```python
from build123d import *

# Parameters (mm, degrees)
EXTRUDE_1_DEPTH     = 3
EXTRUDE_2_DEPTH     = 5.8
SKETCH_3_W          = 1.5
SKETCH_3_H          = 2
SKETCH_3_R          = 0.85
EXTRUDE_3_DEPTH     = 3
CUT_EXTRUDE_1_DEPTH = 8.8


with BuildPart() as part:
    # 草图1 → 凸台-拉伸1 (new body)
    with BuildSketch(Plane.XY):
        Polygon((0, 0), (-28.5, 0), (-28.5, 15), (-8.5, 15), (-8.5, 24.333), (0, 24.333), align=None)
    extrude(amount=EXTRUDE_1_DEPTH)

    # 草图2 → 凸台-拉伸2 (add)
    with BuildSketch(Plane.XY.offset(3)):
        Polygon((-12, 15), (-9.228718708, 10.2), (0, 10.2), (0, 0), (-28.5, 0), (-28.5, 15), align=None)
    extrude(amount=EXTRUDE_2_DEPTH)

    # 草图3 → 凸台-拉伸3 (add)
    with BuildSketch(Plane.XY.offset(3)):
        with Locations((-0.75, 19.6)):
            Rectangle(SKETCH_3_W, SKETCH_3_H)
        with Locations((-0.75, 14.5)):
            Rectangle(SKETCH_3_W, SKETCH_3_H)
        with Locations(Location((-3.5, 13.8, 0), (0, 0, 180))):
            Circle(SKETCH_3_R)
        with Locations(Location((-3.5, 20.3, 0), (0, 0, 180))):
            Circle(SKETCH_3_R)
    extrude(amount=EXTRUDE_3_DEPTH)

    # 草图5 → 切除-拉伸1 (cut)
    with BuildSketch(Plane.XY.offset(8.8)):
        with BuildLine():
            ThreePointArc((-20.5, 7.5), (-22.5, 9.5), (-24.5, 7.5))
            Line((-24.5, 7.5), (-20.5, 7.5))
        make_face()
        with BuildLine():
            Line((-20.5, 7.5), (-24.5, 7.5))
            ThreePointArc((-24.5, 7.5), (-22.5, 5.5), (-20.5, 7.5))
        make_face()
        with BuildLine():
            ThreePointArc((-10.5, 7.5), (-12.5, 9.5), (-14.5, 7.5))
            Line((-14.5, 7.5), (-10.5, 7.5))
        make_face()
        with BuildLine():
            Line((-10.5, 7.5), (-14.5, 7.5))
            ThreePointArc((-14.5, 7.5), (-12.5, 5.5), (-10.5, 7.5))
        make_face()
    extrude(amount=-CUT_EXTRUDE_1_DEPTH, mode=Mode.SUBTRACT)


solid = part.part
```
Work out the finished part from the listing and answer in its coordinate system (mm). A direction names the side the tool comes from. Give positions to 0.01 mm unless a question says otherwise; leave off trailing zeros. Write each loop counter-clockwise with the first axis right and the second up, starting at its lowest first coordinate (ties: lowest second). Pieces come first, ordered by that corner, then holes.
(1) Straight lines are drawn through the part: line 1 (X direction, y = 7.5, z = 3.5); line 2 (Y direction, x = -12.5, z = 4.75); line 3 (X direction, y = 6.75, z = 3). For each, find the intervals that lie inside material, in ascending order.
Final values:
line 1: x = -28.5 to -24.5, -20.5 to -14.5, -10.5 to 0
line 2: y = 0 to 5.5, 9.5 to 15
line 3: x = -28.5 to -24.35, -20.65 to -14.35, -10.65 to 0
(2) Flat-ended cylindrical pins translate along their axes: pin 1 Ø2 at (x, y) = (-22, 5) entering from -Z; pin 2 Ø2.5 at (x, z) = (-19.5, 5.5) entering from +Y; pin 3 Ø0.8 at (x, z) = (-1, 4.5) entering from +Y; pin 4 Ø1.2 at (x, y) = (-0.5, 15) entering from +Z. Find the tip coordinate at first contact, or state that the pin passes through.
Final values:
pin 1: stops at z = 0
pin 2: stops at y = 15
pin 3: stops at y = 20.6
pin 4: stops at z = 6
(3) The part is cut by section D-D on y = 7. Write down the section's boundary in (x, z).
Final values:
outline: (-28.5, 0) - (-24.44, 0) - (-24.44, 8.8) - (-28.5, 8.8) - close; (-20.56, 0) - (-14.44, 0) - (-14.44, 8.8) - (-20.56, 8.8) - close; (-10.56, 0) - (0, 0) - (0, 8.8) - (-10.56, 8.8) - close
(4) The part is cut by section B-B on x = -12.5. Write down the section's boundary in (y, z).
Final values:
outline: (0, 0) - (5.5, 0) - (5.5, 8.8) - (0, 8.8) - close; (9.5, 0) - (15, 0) - (15, 8.8) - (9.5, 8.8) - close
(5) The part is cut by section C-C on z = 7. Write down the section's boundary in (x, y).
Final values:
outline: (-28.5, 0) - (0, 0) - (0, 10.2) - (-9.23, 10.2) - (-12, 15) - (-28.5, 15) - close; hole circle Ø4 at (-22.5, 7.5); hole circle Ø4 at (-12.5, 7.5)
(6) The mould has two halves that part along X. Classify faces 1 (the flat face through (-5, 17, 3)), 2 (the cylindrical face through (-21.026, 6.148, 4.462)), 3 (the flat face through (-3, 14, 6)), 4 (the flat face through (-8.5, 20, 1)): pulls with the +X half, pulls with the -X half, needs draft (parallel to the pull), parting line crosses it, or undercut.
Final values:
face 1: undercut
face 2: undercut
face 3: needs draft
face 4: pulls with the -X half
(7) Which of the six approach directions +Z, -Z, +X, -X, +Y, -Y give full straight-line access (tool end or side, diameter ignored) to faces 5 (the flat face through (-1, 13.5, 4)), 6 (the flat face through (-1, 20, 6)), 7 (the flat face through (-1.5, 20, 4)), 8 (the flat face through (-1, 15, 6)), 9 (the flat face through (-1, 18.6, 4))?
Final values:
face 5: +Z, +X
face 6: +Z, +X, -X, +Y
face 7: +Z, +Y
face 8: +Z, +X, +Y
face 9: +Z, +X, -X
(8) The part is cut by section A-A on z = 3.5. Write down the section's boundary in (x, y).
Final values:
outline: (-28.5, 0) - (0, 0) - (0, 10.2) - (-9.23, 10.2) - (-12, 15) - (-28.5, 15) - close; circle Ø1.7 at (-3.5, 13.8); circle Ø1.7 at (-3.5, 20.3); (-1.5, 13.5) - (0, 13.5) - (0, 15.5) - (-1.5, 15.5) - close; (-1.5, 18.6) - (0, 18.6) - (0, 20.6) - (-1.5, 20.6) - close; hole circle Ø4 at (-22.5, 7.5); hole circle Ø4 at (-12.5, 7.5)
